Autodesk Inventor part; units mm, degrees
ref_plane "YZ Plane" through (0, 0, 0) normal (1, 0, 0) x (0, 1, 0)
ref_plane "XZ Plane" through (0, 0, 0) normal (0, 1, 0) x (-1, 0, 0)
ref_plane "XY Plane" through (0, 0, 0) normal (0, 0, 1) x (1, 0, 0)
sketch "Sketch1" plane through (0, 0, 0) normal (0, 0, 1) x (1, 0, 0)
  line L0 (27.361, 9.329) -> (25.8429, 13.5)
  line L1 (25.8429, 13.5) -> (24.1571, 13.5)
  line L2 (24.1571, 13.5) -> (22.639, 9.329)
  arc A0 (22.1692, 9) -> (22.639, 9.329) centre (22.1692, 9.5) ccw
  line L3 (22.1692, 9) -> (0, 9)
  line L4 (0, 9) -> (0, 0)
  line L5 (0, 0) -> (175.6637, 0)
  line L6 (175.6637, 0) -> (175.6637, 9)
  line L7 (175.6637, 9) -> (153.4945, 9)
  arc A1 (153.0247, 9.329) -> (153.4945, 9) centre (153.4945, 9.5) ccw
  line L8 (153.0247, 9.329) -> (151.5066, 13.5)
  line L9 (151.5066, 13.5) -> (149.8209, 13.5)
  line L10 (149.8209, 13.5) -> (148.3027, 9.329)
  arc A2 (147.8329, 9) -> (148.3027, 9.329) centre (147.8329, 9.5) ccw
  line L11 (147.8329, 9) -> (147.2113, 9)
  arc A3 (146.7415, 9.329) -> (147.2113, 9) centre (147.2113, 9.5) ccw
  line L12 (146.7415, 9.329) -> (145.2234, 13.5)
  line L13 (145.2234, 13.5) -> (143.5377, 13.5)
  line L14 (143.5377, 13.5) -> (142.0195, 9.329)
  arc A4 (141.5497, 9) -> (142.0195, 9.329) centre (141.5497, 9.5) ccw
  line L15 (141.5497, 9) -> (140.9282, 9)
  arc A5 (140.4583, 9.329) -> (140.9282, 9) centre (140.9282, 9.5) ccw
  line L16 (140.4583, 9.329) -> (138.9402, 13.5)
  line L17 (138.9402, 13.5) -> (137.2545, 13.5)
  line L18 (137.2545, 13.5) -> (135.7364, 9.329)
  arc A6 (135.2665, 9) -> (135.7364, 9.329) centre (135.2665, 9.5) ccw
  line L19 (135.2665, 9) -> (134.645, 9)
  arc A7 (134.1751, 9.329) -> (134.645, 9) centre (134.645, 9.5) ccw
  line L20 (134.1751, 9.329) -> (132.657, 13.5)
  line L21 (132.657, 13.5) -> (130.9713, 13.5)
  line L22 (130.9713, 13.5) -> (129.4532, 9.329)
  arc A8 (128.9833, 9) -> (129.4532, 9.329) centre (128.9833, 9.5) ccw
  line L23 (128.9833, 9) -> (128.3618, 9)
  arc A9 (127.8919, 9.329) -> (128.3618, 9) centre (128.3618, 9.5) ccw
  line L24 (127.8919, 9.329) -> (126.3738, 13.5)
  line L25 (126.3738, 13.5) -> (124.6881, 13.5)
  line L26 (124.6881, 13.5) -> (123.17, 9.329)
  arc A10 (122.7001, 9) -> (123.17, 9.329) centre (122.7001, 9.5) ccw
  line L27 (122.7001, 9) -> (122.0786, 9)
  arc A11 (121.6088, 9.329) -> (122.0786, 9) centre (122.0786, 9.5) ccw
  line L28 (121.6088, 9.329) -> (120.0906, 13.5)
  line L29 (120.0906, 13.5) -> (118.4049, 13.5)
  line L30 (118.4049, 13.5) -> (116.8868, 9.329)
  arc A12 (116.417, 9) -> (116.8868, 9.329) centre (116.417, 9.5) ccw
  line L31 (116.417, 9) -> (115.7954, 9)
  arc A13 (115.3256, 9.329) -> (115.7954, 9) centre (115.7954, 9.5) ccw
  line L32 (115.3256, 9.329) -> (113.8075, 13.5)
  line L33 (113.8075, 13.5) -> (112.1217, 13.5)
  line L34 (112.1217, 13.5) -> (110.6036, 9.329)
  arc A14 (110.1338, 9) -> (110.6036, 9.329) centre (110.1338, 9.5) ccw
  line L35 (110.1338, 9) -> (109.5122, 9)
  arc A15 (109.0424, 9.329) -> (109.5122, 9) centre (109.5122, 9.5) ccw
  line L36 (109.0424, 9.329) -> (107.5243, 13.5)
  line L37 (107.5243, 13.5) -> (105.8386, 13.5)
  line L38 (105.8386, 13.5) -> (104.3204, 9.329)
  arc A16 (103.8506, 9) -> (104.3204, 9.329) centre (103.8506, 9.5) ccw
  line L39 (103.8506, 9) -> (103.229, 9)
  arc A17 (102.7592, 9.329) -> (103.229, 9) centre (103.229, 9.5) ccw
  line L40 (102.7592, 9.329) -> (101.2411, 13.5)
  line L41 (101.2411, 13.5) -> (99.5554, 13.5)
  line L42 (99.5554, 13.5) -> (98.0372, 9.329)
  arc A18 (97.5674, 9) -> (98.0372, 9.329) centre (97.5674, 9.5) ccw
  line L43 (97.5674, 9) -> (96.9459, 9)
  arc A19 (96.476, 9.329) -> (96.9459, 9) centre (96.9459, 9.5) ccw
  line L44 (96.476, 9.329) -> (94.9579, 13.5)
  line L45 (94.9579, 13.5) -> (93.2722, 13.5)
  line L46 (93.2722, 13.5) -> (91.7541, 9.329)
  arc A20 (91.2842, 9) -> (91.7541, 9.329) centre (91.2842, 9.5) ccw
  line L47 (91.2842, 9) -> (90.6627, 9)
  arc A21 (90.1928, 9.329) -> (90.6627, 9) centre (90.6627, 9.5) ccw
  line L48 (90.1928, 9.329) -> (88.6747, 13.5)
  line L49 (88.6747, 13.5) -> (86.989, 13.5)
  line L50 (86.989, 13.5) -> (85.4709, 9.329)
  arc A22 (85.001, 9) -> (85.4709, 9.329) centre (85.001, 9.5) ccw
  line L51 (85.001, 9) -> (84.3795, 9)
  arc A23 (83.9096, 9.329) -> (84.3795, 9) centre (84.3795, 9.5) ccw
  line L52 (83.9096, 9.329) -> (82.3915, 13.5)
  line L53 (82.3915, 13.5) -> (80.7058, 13.5)
  line L54 (80.7058, 13.5) -> (79.1877, 9.329)
  arc A24 (78.7178, 9) -> (79.1877, 9.329) centre (78.7178, 9.5) ccw
  line L55 (78.7178, 9) -> (78.0963, 9)
  arc A25 (77.6265, 9.329) -> (78.0963, 9) centre (78.0963, 9.5) ccw
  line L56 (77.6265, 9.329) -> (76.1083, 13.5)
  line L57 (76.1083, 13.5) -> (74.4226, 13.5)
  line L58 (74.4226, 13.5) -> (72.9045, 9.329)
  arc A26 (72.4347, 9) -> (72.9045, 9.329) centre (72.4347, 9.5) ccw
  line L59 (72.4347, 9) -> (71.8131, 9)
  arc A27 (71.3433, 9.329) -> (71.8131, 9) centre (71.8131, 9.5) ccw
  line L60 (71.3433, 9.329) -> (69.8252, 13.5)
  line L61 (69.8252, 13.5) -> (68.1394, 13.5)
  line L62 (68.1394, 13.5) -> (66.6213, 9.329)
  arc A28 (66.1515, 9) -> (66.6213, 9.329) centre (66.1515, 9.5) ccw
  line L63 (66.1515, 9) -> (65.5299, 9)
  arc A29 (65.0601, 9.329) -> (65.5299, 9) centre (65.5299, 9.5) ccw
  line L64 (65.0601, 9.329) -> (63.542, 13.5)
  line L65 (63.542, 13.5) -> (61.8563, 13.5)
  line L66 (61.8563, 13.5) -> (60.3381, 9.329)
  arc A30 (59.8683, 9) -> (60.3381, 9.329) centre (59.8683, 9.5) ccw
  line L67 (59.8683, 9) -> (59.2468, 9)
  arc A31 (58.7769, 9.329) -> (59.2468, 9) centre (59.2468, 9.5) ccw
  line L68 (58.7769, 9.329) -> (57.2588, 13.5)
  line L69 (57.2588, 13.5) -> (55.5731, 13.5)
  line L70 (55.5731, 13.5) -> (54.0549, 9.329)
  arc A32 (53.5851, 9) -> (54.0549, 9.329) centre (53.5851, 9.5) ccw
  line L71 (53.5851, 9) -> (52.9636, 9)
  arc A33 (52.4937, 9.329) -> (52.9636, 9) centre (52.9636, 9.5) ccw
  line L72 (52.4937, 9.329) -> (50.9756, 13.5)
  line L73 (50.9756, 13.5) -> (49.2899, 13.5)
  line L74 (49.2899, 13.5) -> (47.7718, 9.329)
  arc A34 (47.3019, 9) -> (47.7718, 9.329) centre (47.3019, 9.5) ccw
  line L75 (47.3019, 9) -> (46.6804, 9)
  arc A35 (46.2105, 9.329) -> (46.6804, 9) centre (46.6804, 9.5) ccw
  line L76 (46.2105, 9.329) -> (44.6924, 13.5)
  line L77 (44.6924, 13.5) -> (43.0067, 13.5)
  line L78 (43.0067, 13.5) -> (41.4886, 9.329)
  arc A36 (41.0187, 9) -> (41.4886, 9.329) centre (41.0187, 9.5) ccw
  line L79 (41.0187, 9) -> (40.3972, 9)
  arc A37 (39.9273, 9.329) -> (40.3972, 9) centre (40.3972, 9.5) ccw
  line L80 (39.9273, 9.329) -> (38.4092, 13.5)
  line L81 (38.4092, 13.5) -> (36.7235, 13.5)
  line L82 (36.7235, 13.5) -> (35.2054, 9.329)
  arc A38 (34.7355, 9) -> (35.2054, 9.329) centre (34.7355, 9.5) ccw
  line L83 (34.7355, 9) -> (34.114, 9)
  arc A39 (33.6442, 9.329) -> (34.114, 9) centre (34.114, 9.5) ccw
  line L84 (33.6442, 9.329) -> (32.126, 13.5)
  line L85 (32.126, 13.5) -> (30.4403, 13.5)
  line L86 (30.4403, 13.5) -> (28.9222, 9.329)
  arc A40 (28.4524, 9) -> (28.9222, 9.329) centre (28.4524, 9.5) ccw
  line L87 (28.4524, 9) -> (27.8308, 9)
  arc A41 (27.361, 9.329) -> (27.8308, 9) centre (27.8308, 9.5) ccw
  point P0 (87.8319, 5)
extrude "Extrusion1" add sketch "Sketch1" along normal blind 12.7
sketch "Sketch2" plane through (0, 0, 12.7) normal (0, 0, 1) x (1, 0, 0)
  line L0 (0, 9) -> (22.1692, 9)
  line L1 (175.6637, 9) -> (153.4945, 9)
  line L2 (0, 9) -> (175.6637, 9)
  point P0 (0, 0)
sketch "Sketch3" plane through (0, 0, 12.7) normal (0, 0, 1) x (1, 0, 0)
  line L0 (22.639, 9.329) -> (24.1571, 13.5)
  line L1 (175.6637, 0) -> (0, 0)
  line L2 (22.639, 9.329) -> (0, 9.329)
  line L3 (0, 9.329) -> (0, 0)
  line L4 (0, 0) -> (22.639, 0)
  line L5 (22.639, 0) -> (22.639, 9.329)
  line L6 (22.639, 0) -> (98.839, 0)
  line L7 (98.0372, 13.6919) -> (175.6637, 13.6919)
  line L8 (175.6637, 13.6919) -> (175.6637, 0)
  line L9 (175.6637, 0) -> (98.0372, 0)
  line L10 (98.0372, 0) -> (98.0372, 13.6919)
  line L11 (22.639, 0) -> (98.0372, 0)
  line L12 (98.0372, 0) -> (98.0372, 6.846)
  line L13 (98.0372, 6.846) -> (22.639, 6.846)
  line L14 (22.639, 6.846) -> (22.639, 0)
  dimension "d3" = 13.6919
  dimension "d4" = 77.6265
  dimension "d5" = 74.7953
extrude "Extrusion2" cut sketch "Sketch3" against normal blind 25.4
properties part number "Rack"
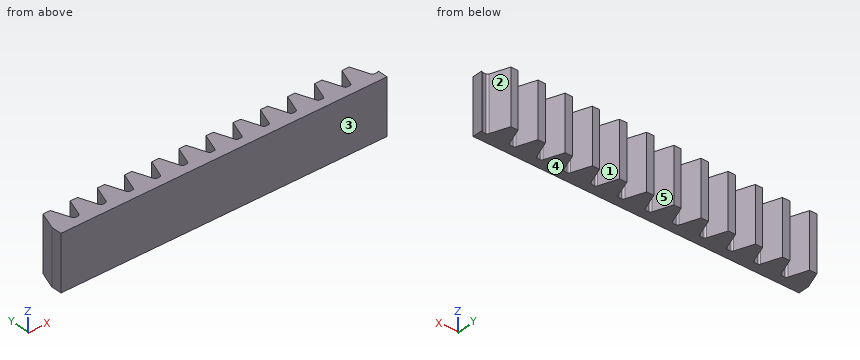
Part model, mm, in its own coordinate system. Face numbers are marked on the shaded views. A direction names the side the tool comes from. Give positions to 0.01 mm unless a question says otherwise; leave off trailing zeros. Use a Markdown table: item, result. Add a question column.
(1) 3-axis set-ups, long thin cutter, end or side, ignore diameter. For the marked faces 4 and 5: which of +Z, -Z, +X, -X, +Y, -Y reach the whole face in a straight line?
(2) Saw through at A-A, the plane y = 12.5. Give the number of separate pieces and of enclosed holes in the cut face, and give its area (3 significant figures).
(3) Drop flat-ended pins along their axis: P1, Ø2, axis at y = 11.5, z = 7.5, coming from the -X side; P2, Ø0.5, axis at x = 97.5, z = 4, coming from the +Y side; P3, Ø0.7, axis at x = 53, z = 6.5, coming from the +Y side. Give the stop position or say it passes through.
(4) Probe line 1 along Y through (x, z) = (28, 7.75); line 2 along Y through (x, z) = (40, 9.5). List the from-to ranges inside material, lowest first. Write a range as [from, to].
(5) Mould opens along X. For the marked faces 1, 2 and 3 say: +X half, -X half, draft (parallel to the pull), parting line (faces both ways), or undercut.
Answer key:
| question | item | result |
|---|---|---|
| 1 | face 4 | -Z, +X, -X, +Y, -Y |
| 1 | face 5 | +Z, -Z, +Y |
| 2 | separate pieces | 12 |
| 2 | enclosed holes | 0 |
| 2 | area | 368 mm^2 |
| 3 | P1 | x = 23.07 |
| 3 | P2 | y = 9.03 |
| 3 | P3 | y = 9.11 |
| 4 | line 1 | [6.85, 9] |
| 4 | line 2 | [6.85, 9.2] |
| 5 | face 1 | undercut |
| 5 | face 2 | +X half |
| 5 | face 3 | draft |
